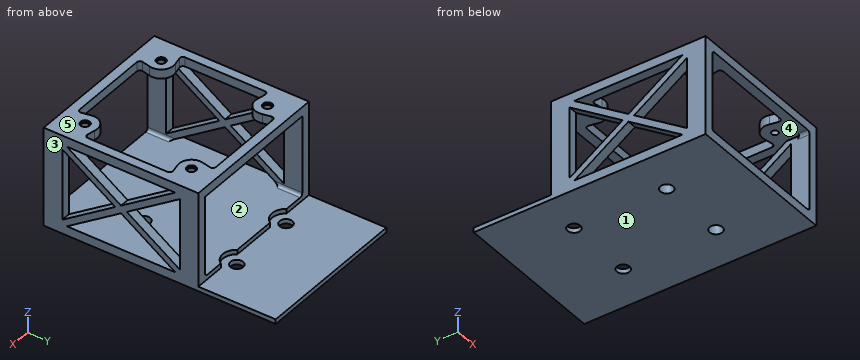
Autodesk Fusion 360 part; units mm, degrees
sketch "Esboço1" plane through (0, 0, 0) normal (0, 0, 1) x (1, 0, 0)
  line L0 (-20, 37.5) -> (20, 37.5)
  line L1 (25, 32.5) -> (25, -37.5)
  line L2 (25, -37.5) -> (-25, -37.5)
  line L3 (-25, -37.5) -> (-25, 32.5)
  line L4 (-25, 37.5) -> (25, -37.5) construction
  line L5 (25, 37.5) -> (-25, -37.5) construction
  line L6 (-25, 32.5) -> (-25, 37.5)
  line L7 (-20, 37.5) -> (-25, 37.5)
  line L8 (20, 37.5) -> (25, 37.5)
  line L9 (25, 32.5) -> (25, 37.5)
  dimension "d1" = 50
  dimension "d2" = 75
extrude "Extrusão1" add sketch "Esboço1" along normal blind 32
sketch "Esboço2" plane through (0, 0, 32) normal (0, 0, 1) x (-1, 0, 0)
  line L0 (-25, 37.5) -> (-25, -37.5)
  line L1 (-25, -37.5) -> (25, -37.5)
  line L2 (25, -37.5) -> (25, 37.5)
  line L3 (25, 37.5) -> (-25, 37.5)
  circle A0 centre (11.137, -15) radius 2.05
  circle A1 centre (-11.137, -15) radius 2.05
  circle A2 centre (11.137, 15) radius 2.05
  circle A3 centre (-11.137, 15) radius 2.05
  dimension "d6" = 4.1
  dimension "d7" = 4.1
  dimension "d8" = 4.1
  dimension "d9" = 4.1
  dimension "d10" = 22.274
  dimension "d11" = 13.863
  dimension "d12" = 13.863
  dimension "d13" = 22.274
  dimension "d14" = 30
  dimension "d15" = 22.5
extrude "Extrusão2" cut sketch "Esboço2" against normal blind 45 contours A0 | A1 | A2 | A3
ref_plane "Plano de trabalho3" through (0, 47.5, 16) normal (0, 1, 0) x (-1, 0, 0)
sketch "Esboço9" plane through (0, 47.5, 0) normal (0, 1, 0) x (-1, 0, 0)
  line L0 (-25, 0) -> (25, 0)
  line L1 (25, 0) -> (25, 32)
  line L2 (25, 32) -> (-25, 32)
  line L3 (-25, 32) -> (-25, 0)
  line L4 (16.763, 29) -> (-16.763, 29)
  line L5 (-22, 25.7693) -> (-22, 6.2307)
  line L6 (-16.763, 3) -> (16.763, 3)
  line L7 (21, 3) -> (-21, 3)
  line L8 (-22, 4) -> (-22, 28)
  line L9 (-21, 29) -> (21, 29)
  line L10 (22, 28) -> (22, 4)
  arc A0 (-21, 29) -> (-22, 28) centre (-21, 28) ccw
  arc A1 (22, 28) -> (21, 29) centre (21, 28) ccw
  arc A2 (21, 3) -> (22, 4) centre (21, 4) ccw
  arc A3 (-22, 4) -> (-21, 3) centre (-21, 4) ccw
  line L11 (-25, 0) -> (25, 0)
  line L12 (25, 0) -> (25, 32)
  line L13 (25, 32) -> (-25, 32)
  line L14 (-25, 32) -> (-25, 0)
  dimension "d156" = 1
extrude "Extrusão9" cut sketch "Esboço9" against normal blind 96 contours L4 L5 L6 L7 L8 L9 L10 A0 A1 A2 A3
sketch "Esboço12" plane through (0, 0, 32) normal (0, 0, 1) x (-1, 0, 0)
  circle A0 centre (11.137, -15) radius 2.05
  circle A1 centre (11.137, 15) radius 2.05
  circle A2 centre (-11.137, -15) radius 2.05
  circle A3 centre (-11.137, 15) radius 2.05
  line L0 (-25, 37.5) -> (-25, -37.5)
  line L1 (-25, -37.5) -> (25, -37.5)
  line L2 (25, -37.5) -> (25, 37.5)
  line L3 (25, 37.5) -> (-25, 37.5)
  line L4 (21, 34.5) -> (-21, 34.5)
  line L5 (-22, 33.5) -> (-22, -33.5)
  line L6 (-21, -34.5) -> (21, -34.5)
  line L7 (22, -33.5) -> (22, 33.5)
  line L8 (22, 34.5) -> (-22, -34.5) construction
  line L9 (-22, 34.5) -> (22, -34.5) construction
  arc A4 (-21, 34.5) -> (-22, 33.5) centre (-21, 33.5) ccw
  arc A5 (22, 33.5) -> (21, 34.5) centre (21, 33.5) ccw
  arc A6 (21, -34.5) -> (22, -33.5) centre (21, -33.5) ccw
  arc A7 (-22, -33.5) -> (-21, -34.5) centre (-21, -33.5) ccw
  dimension "d118" = 44
  dimension "d119" = 69
  dimension "d120" = 1
extrude "Extrusão13" cut sketch "Esboço12" against normal blind 5 contours L4 L5 L6 L7 A4 A5 A6 A7
sketch "Esboço13" plane through (0, 0, 32) normal (0, 0, 1) x (-1, 0, 0)
  line L0 (21, -34.5) -> (-21, -34.5)
  arc A0 (-22, -33.5) -> (-21, -34.5) centre (-21, -33.5) ccw
  line L1 (-22, -33.5) -> (-22, 33.5)
  arc A1 (-21, 34.5) -> (-22, 33.5) centre (-21, 33.5) ccw
  line L2 (-21, 34.5) -> (21, 34.5)
  arc A2 (22, 33.5) -> (21, 34.5) centre (21, 33.5) ccw
  line L3 (22, 33.5) -> (22, -33.5)
  arc A3 (21, -34.5) -> (22, -33.5) centre (21, -33.5) ccw
  line L4 (-25, 37.5) -> (-25, -37.5)
  line L5 (-25, -37.5) -> (25, -37.5)
  line L6 (25, -37.5) -> (25, 37.5)
  line L7 (25, 37.5) -> (-25, 37.5)
  circle A4 centre (-17.2, 29.7) radius 1.05
  line L8 (-13.8524, -8.3) -> (-13.2808, -5.5)
  circle A5 centre (-17.2, 29.7) radius 4
  arc A6 (-22, -0.3726) -> (-20.8, -1.3524) centre (-21, -0.3726) ccw
  circle A7 centre (-17.2, -4.7) radius 4
  line L9 (20.8, -1.3524) -> (18, -0.7808)
  line L10 (-22, 25.3726) -> (-22, -0.3726)
  line L11 (12.8726, 34.5) -> (-12.8726, 34.5)
  arc A8 (13.8524, 33.3) -> (12.8726, 34.5) centre (12.8726, 33.5) ccw
  line L12 (20.8, 26.3524) -> (18, 25.7808)
  arc A9 (12.8726, -9.5) -> (13.8524, -8.3) centre (12.8726, -8.5) ccw
  circle A10 centre (17.2, 29.7) radius 4
  line L13 (-20.8, -1.3524) -> (-18, -0.7808)
  arc A11 (25, 32.5) -> (20, 37.5) centre (20, 32.5) ccw
  circle A12 centre (17.2, -4.7) radius 1.05
  line L14 (0, -15) -> (0, 40)
  line L15 (-13.8524, 33.3) -> (-13.2808, 30.5)
  line L16 (-25, 32.5) -> (-25, -17.5)
  line L17 (-12.8726, -9.5) -> (12.8726, -9.5)
  line L18 (-18.25, 30.75) -> (18.25, -5.75) construction
  line L19 (-22, 34.5) -> (22, -9.5) construction
  line L20 (-18.25, -5.75) -> (18.25, -5.75)
  line L21 (22, 34.5) -> (-22, -9.5) construction
  arc A13 (22, 25.3726) -> (20.8, 26.3524) centre (21, 25.3726) ccw
  circle A14 centre (17.2, -4.7) radius 4
  line L22 (22, -0.3726) -> (22, 25.3726)
  line L23 (13.8524, 33.3) -> (13.2808, 30.5)
  circle A15 centre (17.2, 29.7) radius 1.05
  line L24 (18.25, -5.75) -> (18.25, 30.75)
  line L25 (18.25, 30.75) -> (-18.25, 30.75)
  line L26 (18.25, 30.75) -> (-18.25, -5.75) construction
  line L27 (-25, -17.5) -> (25, -17.5)
  arc A16 (-13.8524, -8.3) -> (-12.8726, -9.5) centre (-12.8726, -8.5) ccw
  line L28 (13.8524, -8.3) -> (13.2808, -5.5)
  arc A17 (-20, 37.5) -> (-25, 32.5) centre (-20, 32.5) ccw
  line L29 (25, -17.5) -> (25, 32.5)
  circle A18 centre (-17.2, -4.7) radius 1.05
  line L30 (-20.8, 26.3524) -> (-18, 25.7808)
  line L31 (-18.25, 30.75) -> (-18.25, -5.75)
  arc A19 (20.8, -1.3524) -> (22, -0.3726) centre (21, -0.3726) ccw
  arc A20 (-20.8, 26.3524) -> (-22, 25.3726) centre (-21, 25.3726) ccw
  arc A21 (-12.8726, 34.5) -> (-13.8524, 33.3) centre (-12.8726, 33.5) ccw
  line L32 (44.2599, -12.5) -> (-40.6438, -12.5)
  point P0 (22, -1.5973)
  point P1 (14.0973, -9.5)
  point P2 (-22, 26.5973)
  point P3 (22, 26.5973)
  point P4 (14.0973, 34.5)
  point P5 (-22, -1.5973)
  point P6 (-14.0973, -9.5)
  point P7 (0, 12.5)
  point P8 (0, -15)
  point P9 (0, 12.5)
  point P10 (-14.0973, 34.5)
  dimension "d123" = 36.5
  dimension "d124" = 36.5
  dimension "d125" = 2.1
  dimension "d126" = 2.1
  dimension "d127" = 2.1
  dimension "d128" = 2.1
  dimension "d129" = 44
  dimension "d130" = 44
  dimension "d131" = 8
  dimension "d132" = 8
  dimension "d133" = 8
  dimension "d134" = 8
  dimension "d135" = 4
  dimension "d136" = 4
  dimension "d137" = 4
  dimension "d138" = 4
  dimension "d139" = 4
  dimension "d140" = 4
  dimension "d141" = 4
  dimension "d142" = 4
  dimension "d143" = 1
  dimension "d144" = 3
  dimension "d145" = 3
extrude "Extrusão14" add sketch "Esboço13" against normal blind 3 contours L3 L9 A9 L14 L17 L20 A14 L24 L28 A19 L32 | L2 A2 L3 L6 L7 L11 A11 L14 L22 L29 L32 | L1 A1 L2 L4 L7 L10 L11 L14 L16 A17 L32 | L1 L8 A6 A7 L13 L14 L17 L20 A16 L31 L32 | L2 A2 L3 A8 L12 A10 A13 L23 L24 L25 | L1 A1 L2 A5 L15 L25 L30 L31 A20 A21 | A12 L20 A14 L24 | L20 A14 L24 | A7 L20 A18 L31 | A7 L20 L31 | A10 A15 L24 L25 | A10 L24 L25 | A12 L20 L24 | A4 A5 L25 L31 | A5 L25 L31 | L20 A18 L31 | A15 L24 L25 | A4 L25 L31
sketch "Esboço14" plane through (0, 0, 32) normal (0, 0, 1) x (-1, 0, 0)
  line L0 (22, -12.5) -> (22, -33.5)
  arc A0 (21, -34.5) -> (22, -33.5) centre (21, -33.5) ccw
  line L1 (21, -34.5) -> (-21, -34.5)
  arc A1 (-22, -33.5) -> (-21, -34.5) centre (-21, -33.5) ccw
  line L2 (-22, -33.5) -> (-22, -12.5)
  line L3 (-22, -12.5) -> (22, -12.5)
  circle A2 centre (17.2, -4.7) radius 1.05
  circle A3 centre (-17.2, -4.7) radius 1.05
  circle A4 centre (17.2, 29.7) radius 1.05
  circle A5 centre (-17.2, 29.7) radius 1.05
  arc A6 (20.8, -1.3524) -> (22, -0.3726) centre (21, -0.3726) ccw
  line L4 (20.8, -1.3524) -> (18.25, -0.8318)
  line L5 (18.25, -0.8318) -> (18.25, -0.8403)
  arc A7 (18.25, -0.8403) -> (13.3403, -5.75) centre (17.2, -4.7) ccw
  line L6 (13.3403, -5.75) -> (13.3318, -5.75)
  line L7 (13.3318, -5.75) -> (13.8524, -8.3)
  arc A8 (12.8726, -9.5) -> (13.8524, -8.3) centre (12.8726, -8.5) ccw
  line L8 (12.8726, -9.5) -> (-12.8726, -9.5)
  arc A9 (-13.8524, -8.3) -> (-12.8726, -9.5) centre (-12.8726, -8.5) ccw
  line L9 (-13.8524, -8.3) -> (-13.3318, -5.75)
  line L10 (-13.3318, -5.75) -> (-13.3403, -5.75)
  arc A10 (-13.3403, -5.75) -> (-18.25, -0.8403) centre (-17.2, -4.7) ccw
  line L11 (-18.25, -0.8403) -> (-18.25, -0.8318)
  line L12 (-18.25, -0.8318) -> (-20.8, -1.3524)
  arc A11 (-22, -0.3726) -> (-20.8, -1.3524) centre (-21, -0.3726) ccw
  line L13 (-22, -0.3726) -> (-22, 25.3726)
  arc A12 (-20.8, 26.3524) -> (-22, 25.3726) centre (-21, 25.3726) ccw
  line L14 (-20.8, 26.3524) -> (-18.25, 25.8318)
  line L15 (-18.25, 25.8318) -> (-18.25, 25.8403)
  arc A13 (-18.25, 25.8403) -> (-13.3403, 30.75) centre (-17.2, 29.7) ccw
  line L16 (-13.3403, 30.75) -> (-13.3318, 30.75)
  line L17 (-13.3318, 30.75) -> (-13.8524, 33.3)
  arc A14 (-12.8726, 34.5) -> (-13.8524, 33.3) centre (-12.8726, 33.5) ccw
  line L18 (-12.8726, 34.5) -> (12.8726, 34.5)
  arc A15 (13.8524, 33.3) -> (12.8726, 34.5) centre (12.8726, 33.5) ccw
  line L19 (13.8524, 33.3) -> (13.3318, 30.75)
  line L20 (13.3318, 30.75) -> (13.3403, 30.75)
  arc A16 (13.3403, 30.75) -> (18.25, 25.8403) centre (17.2, 29.7) ccw
  line L21 (18.25, 25.8403) -> (18.25, 25.8318)
  line L22 (18.25, 25.8318) -> (20.8, 26.3524)
  arc A17 (22, 25.3726) -> (20.8, 26.3524) centre (21, 25.3726) ccw
  line L23 (22, 25.3726) -> (22, -0.3726)
  line L24 (25, -37.5) -> (25, 37.5)
  line L25 (25, 37.5) -> (-25, 37.5)
  line L26 (-25, 37.5) -> (-25, -37.5)
  line L27 (-25, -37.5) -> (25, -37.5)
  circle A18 centre (17.2, 29.7) radius 1.5
  circle A19 centre (17.2, -4.7) radius 1.5
  circle A20 centre (-17.2, -4.7) radius 1.5
  circle A21 centre (-17.2, 29.7) radius 1.5
  dimension "d150" = 3
  dimension "d151" = 3
  dimension "d152" = 3
  dimension "d153" = 3
extrude "Extrusão15" cut sketch "Esboço14" against normal blind 0.5 contours A18 | A19 | A20 | A21
sketch "Esboço15" plane through (-25, 0, 0) normal (-1, 0, 0) x (0, -1, 0)
  line L0 (37.5, 32) -> (-37.5, 32)
  line L1 (-37.5, 32) -> (-37.5, 0)
  line L2 (-37.5, 0) -> (37.5, 0)
  line L3 (37.5, 0) -> (37.5, 32)
  line L4 (-9.5, 32) -> (34.5, 32)
  line L5 (34.5, 32) -> (34.5, 0)
  line L6 (34.5, 0) -> (-9.5, 0)
  line L7 (-9.5, 0) -> (-9.5, 32)
  line L8 (31.5, 29) -> (-6.5, 29)
  line L9 (-6.5, 29) -> (-6.5, 3)
  line L10 (-6.5, 3) -> (31.5, 3)
  line L11 (31.5, 3) -> (31.5, 29)
  line L12 (31.5, 29) -> (-6.5, 3) construction
  line L13 (-6.5, 29) -> (31.5, 3) construction
  circle A0 centre (-6.5, 29) radius 1.5
  circle A1 centre (31.5, 29) radius 1.5
  circle A2 centre (31.5, 3) radius 1.5
  circle A3 centre (-6.5, 3) radius 1.5
  line L14 (-5, 3) -> (31.5, 27.5)
  line L15 (-6.5, 4.5) -> (30, 29)
  line L16 (-5, 29) -> (31.5, 4.5)
  line L17 (30, 3) -> (-6.5, 27.5)
  line L18 (-12.5, 32) -> (-42.5, 32)
  line L19 (-42.5, 32) -> (-42.5, 1.5)
  line L20 (-42.5, 1.5) -> (-12.5, 1.5)
  line L21 (-12.5, 1.5) -> (-12.5, 32)
  point P0 (-9.5, 32)
  point P1 (34.5, 32)
  point P2 (12.5, 16)
  point P3 (-12.5, 32)
  dimension "d158" = 44
  dimension "d159" = 32
  dimension "d160" = 38
  dimension "d162" = 3
  dimension "d163" = 3
  dimension "d164" = 3
  dimension "d165" = 3
  dimension "d172" = 30
  dimension "d173" = 30.5
extrude "Extrusão16" cut sketch "Esboço15" against normal blind 60 contours L0 L1 L18 L20 L21 | L8 L15 L16 | L11 L14 L16 | L9 L15 L17 | L10 L14 L17
sketch "Esboço16" plane through (0, 0, 1.5) normal (0, 0, 1) x (-1, 0, 0)
  line L0 (-25, -12.5) -> (-25, -37.5)
  line L1 (-25, -37.5) -> (25, -37.5)
  line L2 (25, -37.5) -> (25, -12.5)
  line L3 (25, -12.5) -> (-25, -12.5)
  circle A0 centre (-11.137, -15) radius 2.05
  circle A1 centre (11.137, -15) radius 2.05
  circle A2 centre (-11.137, -15) radius 4.5
  circle A3 centre (11.137, -15) radius 4.5
  dimension "d174" = 9
  dimension "d175" = 9
extrude "Extrusão17" cut sketch "Esboço16" along normal blind 3 contours L3 A2 | L3 A3 picked at (-11.703, -11.4131) picked at (10.2449, -11.6515)
Source: CAD feature listing. Evaluate the final solid. Frame: model axes, mm. Face numbers are marked on the shaded views. A direction names the side the tool comes from. Coordinates: 2 decimals unless noted, no trailing zeros. Loops run counter-clockwise (first coordinate to the right, second up) from the corner with the lowest first, then second, coordinate; pieces in that order, holes last. Notation, with made-up numbers: (67, 17.25) - (93, 17.25) arc R13 ccw to (93, 30.25) - close; hole circle Ø9 at (76, 72.25). An arc over 180 degrees is marked (long way). Return JSON: item names as keys, results as strings.
Q1. Access query for the marked faces 4 and 5. Directions: +Z, -Z, +X, -X, +Y, -Y. A direction counts if a zero-diameter tool reaches every point of the face in a straight line with its end or side. Return the directions, or none.
Results:
{"face 4": "none", "face 5": "+Z, +X, -X, +Y, -Y"}
Q2. Contact query for flat-ended pins moving along their axis: P1, Ø6, axis at x = 14, y = -9.5, coming from the +Z side; P2, Ø12, axis at x = -7.5, z = 25.5, coming from the +Y side; P3, Ø13.5, axis at x = -12.5, y = 25, coming from the +Z side. Output: stop coordinate, or through.
Results:
{"P1": "z = 3", "P2": "y = 12.5", "P3": "z = 1.5"}
Q3. Material intervals for line 1 along X through (y, z) = (-15, 1); line 2 along Y through (x, z) = (17.2, 29.8); line 3 along Y through (x, z) = (15, 31), sorted ascending.
Results:
{"line 1": "-25 to -13.19, -9.09 to 9.09, 13.19 to 25", "line 2": "-37.5 to -30.75, -28.65 to -25.7, 0.7 to 3.65, 5.75 to 12.5", "line 3": "-37.5 to -26.36, 1.36 to 12.5"}
Q4. Section C-C, the plane x = 3.5. Return loops of the section in (y, z), plus the area to 4 significant figures.
Results:
{"outline": "(-37.5, 0) - (37.5, 0) - (37.5, 1.5) - (12.5, 1.5) - (12.5, 3) - (-37.5, 3) - close; (-37.5, 29) - (-34.5, 29) - (-34.5, 32) - (-37.5, 32) - close; (9.5, 29) - (12.5, 29) - (12.5, 32) - (9.5, 32) - close", "area": "205.5 mm2"}
Q5. Section B-B, the plane x = -17.2. Give the number of separate pieces and of enclosed holes in the cut face, plus the area to 3 significant figures.
Results:
{"separate pieces": "5", "enclosed holes": "0", "area": "245 mm2"}
Q6. Mould query, pull axis Z, two halves, no side actions, for the marked faces 1, 2 and 3. Classes: released by +Z, released by -Z, zero draft, split by the parting line, or undercut.
Results:
{"face 1": "released by -Z", "face 2": "undercut", "face 3": "zero draft"}
Q7. Section A-A, the plane y = 15. Return loops of the section in (x, z).
Results:
{"outline": "(-25, 0) - (-13.19, 0) - (-13.19, 1.5) - (-25, 1.5) - close; (-9.09, 0) - (9.09, 0) - (9.09, 1.5) - (-9.09, 1.5) - close; (13.19, 0) - (25, 0) - (25, 1.5) - (13.19, 1.5) - close"}
